Check sheet for the modelled part. Datum: model origin and axes. Units: mm. A direction names the side the tool comes from. Round coordinates to 2 decimals unless told otherwise and drop trailing zeros. Write each loop counter-clockwise with the first axis right and the second up, starting at its lowest first coordinate (ties: lowest second). Pieces come first, ordered by that corner, then holes. Notation, with made-up numbers: (54, 3.5) -> (101, 3.5) arc R23 ccw to (101, 38.5) -> close; hole circle Ø1 at (70, 9.5). An arc over 180 degrees is marked (long way). One line per item, written item: value.
Autodesk Inventor part; units mm, degrees
ref_plane "YZ Plane" through (0, 0, 0) normal (1, 0, 0) x (0, 1, 0)
ref_plane "XZ Plane" through (0, 0, 0) normal (0, 1, 0) x (-1, 0, 0)
ref_plane "XY Plane" through (0, 0, 0) normal (0, 0, 1) x (1, 0, 0)
sketch "Sketch1" plane through (0, 0, 0) normal (0, 0, 1) x (1, 0, 0)
  line L0 (0, -5.6) -> (0, 5.6)
  line L1 (2.4, -3.2) -> (2.4, 3.2)
  line L2 (2.4, 3.2) -> (3.2, 3.2)
  line L3 (3.2, 3.2) -> (3.2, 4)
  line L4 (3.2, 4) -> (3.6, 4)
  line L5 (3.6, 4) -> (3.6, -4)
  line L6 (3.6, -4) -> (3.2, -4)
  line L7 (3.2, -4) -> (3.2, -3.2)
  line L8 (3.2, -3.2) -> (2.4, -3.2)
  point P0 (0, 0)
  point P1 (2.4, 0)
  dimension "d0" = 4.8
  dimension "d1" = 8
  dimension "d2" = 6.4
  dimension "d3" = 0.8
  dimension "d4" = 7.2
revolve "Revolution1" add sketch "Sketch1" angle 360 about axis through (0, -10, 0) along (0, 1, 0)
fillet "Fillet1" radius 0.1 2 edges at (-3.6, 4, 0) (-3.6, -4, 0)
equation "\"d0\" = tpd"
equation "\"d1\" = lu"
equation "\"d2\" = tsd"
equation "\"d3\" = tsl"
equation "\"d4\" = tlad"
properties part number "18654-Red" material "ABS Plastic"
Item 1: Sectioned sample at C-C (y = 0). Enter the section's corners in (x, z).
Result set:
outline: circle Ø7.2 at (0, 0); hole circle Ø4.8 at (0, 0)
Item 2: Release check for a two-part mould opening along X. For faces 3 (the cylindrical face through (3.434, -0.055, 1.081)), 4 (the cylindrical face through (-2.539, 3.606, 1.947)) record: pulls with the +X half, pulls with the -X half, needs draft (parallel to the pull), parting line crosses it, or undercut.
Result set:
face 3: parting line crosses it
face 4: undercut
Item 3: Depth check by flat-ended pin: pin 1 (4 mm diameter, centred on x = 0, z = 0, fed in from +Y); pin 2 (3 mm diameter, centred on y = 1.5, z = 0.5, fed in from +X); pin 3 (1.5 mm diameter, centred on x = 1, y = 1.5, fed in from -Z). Enter the tip coordinate at first touch or a pass-through.
Result set:
pin 1: through
pin 2: x = 3.6
pin 3: z = -3.59
Item 4: Sectioned sample at A-A (z = 0). Enter the section's corners in (x, y).
Result set:
outline: (-3.6, -3.9) arc R0.1 ccw to (-3.5, -4) -> (-3.2, -4) -> (-3.2, -3.2) -> (-2.4, -3.2) -> (-2.4, 3.2) -> (-3.2, 3.2) -> (-3.2, 4) -> (-3.5, 4) arc R0.1 ccw to (-3.6, 3.9) -> close; (2.4, -3.2) -> (3.2, -3.2) -> (3.2, -4) -> (3.5, -4) arc R0.1 ccw to (3.6, -3.9) -> (3.6, 3.9) arc R0.1 ccw to (3.5, 4) -> (3.2, 4) -> (3.2, 3.2) -> (2.4, 3.2) -> close
Item 5: Tool access check on faces 1 (the cylindrical face through (1.29, 0.045, -2.024)), 2 (the cylindrical face through (-2.539, -3.594, 1.947)). Record the directions out of +Z, -Z, +X, -X, +Y, -Y that give a thin tool (end or side, any length) a straight path to the whole face; none if there is none.
Result set:
face 1: +Y, -Y
face 2: -Y
Item 6: Material ranges on line 1 along Z through (x, y) = (0, 3.55); line 2 along X through (y, z) = (1.75, 0), recorded low to high.
Result set:
line 1: -3.6 to -3.2, 3.2 to 3.6
line 2: -3.6 to -2.4, 2.4 to 3.6
Item 7: Sectioned sample at B-B (x = 0). Enter the section's corners in (y, z).
Result set:
outline: (-4, -3.5) arc R0.1 ccw to (-3.9, -3.6) -> (3.9, -3.6) arc R0.1 ccw to (4, -3.5) -> (4, -3.2) -> (3.2, -3.2) -> (3.2, -2.4) -> (-3.2, -2.4) -> (-3.2, -3.2) -> (-4, -3.2) -> close; (-4, 3.2) -> (-3.2, 3.2) -> (-3.2, 2.4) -> (3.2, 2.4) -> (3.2, 3.2) -> (4, 3.2) -> (4, 3.5) arc R0.1 ccw to (3.9, 3.6) -> (-3.9, 3.6) arc R0.1 ccw to (-4, 3.5) -> close
